Geometry: final body of the model. Coordinates: model frame, mm. A direction names the side the tool comes from. Round coordinates to 2 decimals unless told otherwise and drop trailing zeros. Loops run counter-clockwise (first coordinate to the right, second up) from the corner with the lowest first, then second, coordinate; pieces in that order, holes last. Notation, with made-up numbers: M -5.75,56.25 L 27.25,56.25 A24 cw 27.25,94.25 Z; hole C 60.5,78 d3. An arc over 180 degrees is marked long. Write each question's results on one line, items separated by ' | '.
```python
from build123d import *

# Parameters (mm, degrees)
SALIENTE_EXTRUIR1_DEPTH = 48
CROQUIS3_W              = 4
CROQUIS3_H              = 5.48
SALIENTE_EXTRUIR3_DEPTH = 15
REDONDEO1_R             = 2


with BuildPart() as part:
    # Croquis1 → Saliente-Extruir1 (new body)
    with BuildSketch(Plane(origin=(0, 0, 0), x_dir=(1, 0, 0), z_dir=(0, 1, 0))):
        Polygon((0, 0), (13, 0), (13, 13), (10, 13), (10, 3), (0, 3), align=None)
    extrude(amount=SALIENTE_EXTRUIR1_DEPTH)

    # Croquis3 → Saliente-Extruir3 (add)
    with BuildSketch(Plane(origin=(0, 48, 0), x_dir=(1, 0, 0), z_dir=(0, 1, 0))):
        with Locations((11, 2.74)):
            Rectangle(CROQUIS3_W, CROQUIS3_H)
    extrude(amount=SALIENTE_EXTRUIR3_DEPTH)

    # Redondeo1
    # the kernel refuses this fillet: 2 mm, written as the material it adds along each edge
    with BuildSketch(Plane(origin=(15, 48, -3), x_dir=(0, -1, 0), z_dir=(-1, 0, 0))) as redondeo1_piece_1_section:
        with BuildLine():
            CenterArc((REDONDEO1_R, -REDONDEO1_R), REDONDEO1_R, 90, 90)
            Line((0, -REDONDEO1_R), (0, 0))
            Line((0, 0), (REDONDEO1_R, 0))
        make_face()
    redondeo1_piece_1 = extrude(amount=6, mode=Mode.PRIVATE)
    redondeo1_piece_1 = split(redondeo1_piece_1, bisect_by=Plane(origin=(13, 47.553264122, -3.446735878), z_dir=(-1, 0, 0)), keep=Keep.TOP, mode=Mode.PRIVATE)
    add(redondeo1_piece_1)
    with BuildSketch(Plane(origin=(10, 48, -5.48), x_dir=(-1, 0, 0), z_dir=(0, 0, 1))) as redondeo1_piece_2:
        with BuildLine():
            CenterArc((2, 1.732050808), REDONDEO1_R, 180, 60)
            Line((0, 1.732050808), (0, 0))
            Line((0, 0), (1, 0))
        make_face()
    extrude(amount=2.48)


solid = part.part
```
1. Section B-B (x = 11.75). Output: boundary loops of the cut face in (y, z), then the cut area to 3 significant figures.
Answer key:
outline: M 0,-13 L 48,-13 L 48,-5.48 L 63,-5.48 L 63,0 L 0,0 Z | area: 706 mm²
2. Access query for faces 1 (the face through (11, 48, -9)), 2 (the face through (4, 48, -2)), 3 (the face through (10, 24, -8)). Directions: +Z, -Z, +X, -X, +Y, -Y. A direction counts if a zero-diameter tool reaches every point of the face in a straight line with its end or side. Return the directions, or none.
Answer key:
face 1: -Z, +X, -X, +Y | face 2: +Z, -Z, -X, +Y | face 3: -Z, -X, -Y
3. Pin query (flat end, axial travel): P1, Ø0.9, axis at x = 11.5, z = -11, coming from the +Y side; P2, Ø4, axis at x = 7, y = 21.5, coming from the -Z side; P3, Ø3, axis at x = 12, y = 58, coming from the -Z side. Return the tip coordinate at first contact, or that it passes through.
Answer key:
P1: stops at y = 48 | P2: stops at z = -3 | P3: stops at z = -5.48
4. Section D-D (z = -8.75). Output: boundary loops of the cut face in (x, y), then the cut area to 3 significant figures.
Answer key:
outline: M 10,0 L 13,0 L 13,48 L 10,48 Z | area: 144 mm²
5. Section C-C (z = -4). Output: boundary loops of the cut face in (x, y), then the cut area to 3 significant figures.
Answer key:
outline: M 9,47.73 L 9.36,47.73 A2 cw 10,46.27 L 10,0 L 13,0 L 13,63 L 9,63 Z | area: 205 mm²
6. Section A-A (y = 26.5). Output: boundary loops of the cut face in (x, z), then the cut area to 3 significant figures.
Answer key:
outline: M 0,-3 L 10,-3 L 10,-13 L 13,-13 L 13,0 L 0,0 Z | area: 69.0 mm²
7. Ray query, probe 1 along Y at (x, z) = (8.5, -1); probe 2 along X at (y, z) = (43, -4); probe 3 along Z at (x, y) = (4.25, 13). Return the intervals inside material, ascending.
Answer key:
probe 1: y = 0 to 48 | probe 2: x = 10 to 13 | probe 3: z = -3 to 0
